from build123d import *

# Parameters (mm, degrees)
SKETCH002_W      = 145
SKETCH002_H      = 94
PAD004_DEPTH     = 6
HOLE_D           = 6.1
HOLE_DEPTH       = 5
HOLE_CSINK_D     = 6.5
HOLE_CSINK_ANGLE = 90
SKETCH013_R      = 15
SKETCH014_R      = 5.75
SKETCH005_R      = 5.75


with BuildPart() as part:
    # Sketch002 → Pad004 (new body)
    with BuildSketch(Plane.XZ.offset(-12.5)):
        with Locations((-27.5, 12)):
            Rectangle(SKETCH002_W, SKETCH002_H)
    extrude(amount=-PAD004_DEPTH)

    # Hole
    with Locations(Plane.XZ.offset(-12.5)):
        with Locations((30, 50)):
            CounterSinkHole(HOLE_D / 2, HOLE_CSINK_D / 2, depth=HOLE_DEPTH, counter_sink_angle=HOLE_CSINK_ANGLE)

    # Sketch013 → AdditiveLoft001 section 0
    with BuildSketch(Plane.XZ.offset(-12.5)):
        with Locations((-80.75, 15)):
            Circle(SKETCH013_R)
    # Sketch014 → AdditiveLoft001 section 1
    with BuildSketch(Plane.XZ.offset(12.5)):
        with Locations((-90, 15)):
            Circle(SKETCH014_R)
    # Sketch005 → AdditiveLoft001 section 2
    with BuildSketch(Plane.XZ.offset(27.5)):
        with Locations((-90, 15)):
            Circle(SKETCH005_R)
    loft(ruled=True)


solid = part.part
Geometry check sheet. Reference: the model listing, model coordinates, mm. A direction names the side the tool comes from. Round coordinates to 2 decimals unless told otherwise and drop trailing zeros. Write each loop counter-clockwise with the first axis right and the second up, starting at its lowest first coordinate (ties: lowest second). Pieces come first, ordered by that corner, then holes.
Item 1: Access from +Z, -Z, +X, -X, +Y, -Y to the whole of each face (thin tool, end or side, straight path). Record for faces 4 (the face through (-90, -27.5, 15)), 5 (the face through (30, 17.5, 50)).
Determined:
face 4: +Z, -Z, +X, -X, -Y
face 5: -Y
Item 2: Section check C-C (y = -14). Record the boundary of the cut face in (x, z), plus the area to 3 significant figures.
Determined:
outline: circle Ø11.5 at (-90, 15)
area: 104 mm2
Item 3: Mould release check, pull along Z, two halves, no side actions. Record for faces 1 (the face through (45, 15, 11)), 2 (the face through (28.593, 15.134, 47.294)), 3 (the face through (-95.744, -20.105, 15.253)): +Z half, -Z half, draft (parallel to the pull), parting line (faces both ways), or undercut.
Determined:
face 1: draft
face 2: undercut
face 3: parting line
Item 4: Go/stop test with flat-tipped pins: pin 1 Ø4 at (x, z) = (-78, -24) entering from -Y; pin 2 Ø3 at (y, z) = (10, 32.5) entering from -X. Record where each tip stops, or that it passes through.
Determined:
pin 1: stops at y = 12.5
pin 2: passes through
Item 5: Material ranges on line 1 along X through (y, z) = (16, 50); line 2 along Z through (x, y) = (30, 14.55); line 3 along Y through (x, z) = (-51, 28), recorded low to high.
Determined:
line 1: x = -100 to 26.95, 33.05 to 45
line 2: z = -35 to 46.95, 53.05 to 59
line 3: y = 12.5 to 18.5
Item 6: Section check D-D (z = -4). Record the boundary of the cut face in (x, y).
Determined:
outline: (-100, 12.5) - (45, 12.5) - (45, 18.5) - (-100, 18.5) - close
Item 7: Section check A-A (x = 30). Record the boundary of the cut face in (y, z), plus the area to 3 significant figures.
Determined:
outline: (12.5, -35) - (18.5, -35) - (18.5, 59) - (12.5, 59) - (12.5, 53.25) - (12.7, 53.05) - (17.5, 53.05) - (17.5, 46.95) - (12.7, 46.95) - (12.5, 46.75) - close
area: 533 mm2
Item 8: Section check B-B (z = 50). Record the boundary of the cut face in (x, y).
Determined:
outline: (-100, 12.5) - (26.75, 12.5) - (26.95, 12.7) - (26.95, 17.5) - (33.05, 17.5) - (33.05, 12.7) - (33.25, 12.5) - (45, 12.5) - (45, 18.5) - (-100, 18.5) - close
